Part model, mm, in its own coordinate system. A direction names the side the tool comes from. Round coordinates to 2 decimals unless told otherwise and drop trailing zeros. Write each loop counter-clockwise with the first axis right and the second up, starting at its lowest first coordinate (ties: lowest second). Pieces come first, ordered by that corner, then holes. Notation, with made-up numbers: M -32,71.25 L -11,71.25 A11 cw -11,86.25 Z; hole C 73.25,-10 d9. An arc over 180 degrees is marked long. Answer as a JSON object with one key per item and string values. Group by question number.
1. Two-plate mould, pull along Y, no slides. Class faces 1 (the face through (28, 4.75, -31)), 2 (the face through (57, 8, -10)), 3 (the face through (11.07, 6.34, -19.08)): +Y half, -Y half, draft (parallel to the pull), parting line (faces both ways), or undercut.
2. Band-saw the part on B-B, the plane z = -17.5. Write the cut outline in (x, y), plus the area to 3 significant figures.
3. Drop flat-ended pins along their axis: pin 1 (2.5 mm diameter, centred on x = 27.52, z = -32.31, fed in from +Y); pin 2 (2 mm diameter, centred on x = 39.5, y = 5.5, fed in from +Z); pin 3 (4 mm diameter, centred on x = 28, z = -31.5, fed in from +Y); pin 4 (2 mm diameter, centred on x = 44, z = -13.5, fed in from +Y). Give the stop position or say it passes through.
4. Band-saw the part on C-C, the plane z = -25. Write the cut outline in (x, y), plus the area to 3 significant figures.
5. Which spindle directions (+Z, -Z, +X, -X, +Y, -Y) get a long thin tool onto all of the face, cutting with end or side? Do faces 4 (the face through (30, 4.75, -18)), 5 (the face through (-1.15, 8.83, -4.93)), 6 (the face through (15.5, 6, -17)), 7 (the face through (28, 12, -35.17)). Say none if no direction does.
6. Drill centre lines: line 1 (X direction, y = 4, z = -27.5); line 2 (X direction, y = 6.5, z = -27.5); line 3 (X direction, y = 4.25, z = -15). Where is each one in solid material? Low to high. Write a range as from..to.
7. Band-saw the part on A-A, the plane x = 8.5. Write the cut outline in (y, z), plus the area to 3 significant figures.
8. Band-saw the part on D-D, the plane x = 54. Write the cut outline in (y, z), plus the area to 3 significant figures.
from build123d import *

# Parameters (mm, degrees)
SKETCH1_W                            = 55
SKETCH1_H                            = 42.17
BOSS_EXTRUDE1_DEPTH                  = 12.5
SKETCH2_W                            = 55
SKETCH2_H                            = 7
BOSS_EXTRUDE2_DEPTH                  = 2.5
SKETCH3_W                            = 16.25
SKETCH3_H                            = 35.17
CUT_EXTRUDE1_DEPTH                   = 7.25
CUT_EXTRUDE2_DEPTH                   = 71.424135777
SKETCH5_R                            = 2.85
SKETCH5_R_2                          = 2.35
CUT_EXTRUDE3_DEPTH                   = 0.5
SKETCH7_R                            = 5
BOSS_EXTRUDE3_DEPTH                  = 4
TAP_DRILL_FOR_10_32_TAP1_D           = 4.0386
TAP_DRILL_FOR_10_32_TAP1_DEPTH       = 4
TAP_DRILL_FOR_10_32_TAP1_CSINK_D     = 5.3086
TAP_DRILL_FOR_10_32_TAP1_CSINK_ANGLE = 90
TAP_DRILL_FOR_10_32_TAP1_TIP         = 1.213317848
SKETCH11_R                           = 1
CUT_EXTRUDE4_DEPTH                   = 71.059770197
TAP_DRILL_FOR_M3X0_5_TAP1_D          = 2.5
SKETCH15_R                           = 1.58
CUT_EXTRUDE5_DEPTH                   = 72.242956845
TAP_DRILL_FOR_M3X0_5_TAP3_D          = 2.5
TAP_DRILL_FOR_M3X0_5_TAP3_DEPTH      = 10
TAP_DRILL_FOR_M3X0_5_TAP3_TIP        = 0.751075774
BOSS_EXTRUDE4_DEPTH                  = 7
BOSS_EXTRUDE5_DEPTH                  = 7
SKETCH24_R                           = 1.58
CUT_EXTRUDE6_DEPTH                   = 10
TAP_DRILL_FOR_M3X0_5_TAP2_D          = 2.5


with BuildPart() as part:
    # Sketch1 → Boss-Extrude1 (new body)
    with BuildSketch(Plane(origin=(0, 0, 0), x_dir=(1, 0, 0), z_dir=(0, 1, 0))):
        with Locations((27.5, 21.085)):
            Rectangle(SKETCH1_W, SKETCH1_H)
    extrude(amount=BOSS_EXTRUDE1_DEPTH)

    # Sketch2 → Boss-Extrude2 (add)
    with BuildSketch(Plane(origin=(0, 12.5, 0), x_dir=(1, 0, 0), z_dir=(0, 1, 0))):
        with Locations((27.5, 38.67)):
            Rectangle(SKETCH2_W, SKETCH2_H)
    extrude(amount=BOSS_EXTRUDE2_DEPTH)

    # Sketch3 → Cut-Extrude1 (cut)
    with BuildSketch(Plane(origin=(0, 12.5, 0), x_dir=(1, 0, 0), z_dir=(0, 1, 0))):
        with Locations((25.465, 17.585)):
            Rectangle(SKETCH3_W, SKETCH3_H)
    extrude(amount=-CUT_EXTRUDE1_DEPTH, mode=Mode.SUBTRACT)

    # Sketch4 → Cut-Extrude2 (cut, through all)
    with BuildSketch(Plane(origin=(0, 12.5, 0), x_dir=(1, 0, 0), z_dir=(0, 1, 0))):
        with BuildLine():
            Line((15.5, 3.917342747), (15.5, 30.917342747))
            ThreePointArc((15.5, 30.917342747), (15.792893219, 31.624449528), (16.5, 31.917342747))
            Line((16.5, 31.917342747), (19.34, 31.917342747))
            ThreePointArc((19.34, 31.917342747), (20.047106781, 31.624449528), (20.34, 30.917342747))
            Line((20.34, 30.917342747), (20.34, 3.917342747))
            ThreePointArc((20.34, 3.917342747), (20.047106781, 3.210235966), (19.34, 2.917342747))
            Line((19.34, 2.917342747), (16.5, 2.917342747))
            ThreePointArc((16.5, 2.917342747), (15.792893219, 3.210235966), (15.5, 3.917342747))
        make_face()
    extrude(amount=-CUT_EXTRUDE2_DEPTH, mode=Mode.SUBTRACT)

    # Sketch5 → Cut-Extrude3 (cut)
    with BuildSketch(Plane(origin=(0, 5.25, 0), x_dir=(1, 0, 0), z_dir=(0, 1, 0))):
        with Locations(Location((24.34, 4.307342747, 0), (0, 0, 270))):
            Circle(SKETCH5_R)
        with Locations(Location((26.34, 11.307342747, 0), (0, 0, 270))):
            Circle(SKETCH5_R)
        with Locations(Location((29.84, 18.307342747, 0), (0, 0, 270))):
            Circle(SKETCH5_R)
        with Locations(Location((23.84, 25.307342747, 0), (0, 0, 270))):
            Circle(SKETCH5_R)
        with Locations(Location((27.52, 32.307342747, 0), (0, 0, 270))):
            Circle(SKETCH5_R_2)
    extrude(amount=-CUT_EXTRUDE3_DEPTH, mode=Mode.SUBTRACT)

    # Sketch7 → Boss-Extrude3 (add)
    with BuildSketch(Plane.XZ):
        with Locations(Location((27.52, -32.307342747, 0), (0, 0, 270))):
            Circle(SKETCH7_R)
    extrude(amount=BOSS_EXTRUDE3_DEPTH)

    # Tap Drill for #10-32 Tap1
    with Locations(Plane(origin=(0, -4, 0), x_dir=(-1, 0, 0), z_dir=(0, -1, 0))):
        with Locations((-27.52, 32.307342747)):
            CounterSinkHole(TAP_DRILL_FOR_10_32_TAP1_D / 2, TAP_DRILL_FOR_10_32_TAP1_CSINK_D / 2, depth=TAP_DRILL_FOR_10_32_TAP1_DEPTH, counter_sink_angle=TAP_DRILL_FOR_10_32_TAP1_CSINK_ANGLE)
            with Locations((0, 0, -(TAP_DRILL_FOR_10_32_TAP1_DEPTH + TAP_DRILL_FOR_10_32_TAP1_TIP / 2))):  # 118° drill point
                Cone(0, TAP_DRILL_FOR_10_32_TAP1_D / 2, TAP_DRILL_FOR_10_32_TAP1_TIP, mode=Mode.SUBTRACT)

    # Sketch11 → Cut-Extrude4 (cut, through all)
    with BuildSketch(Plane(origin=(0, 4.75, 0), x_dir=(1, 0, 0), z_dir=(0, 1, 0))):
        with Locations(Location((27.52, 32.307342747, 0), (0, 0, 270))):
            Circle(SKETCH11_R)
    extrude(amount=-CUT_EXTRUDE4_DEPTH, mode=Mode.SUBTRACT)

    # Tap Drill for M3x0.5 Tap1 (through all)
    with Locations(Plane(origin=(0, 12.5, 0), x_dir=(1, 0, 0), z_dir=(0, 1, 0))):
        with Locations((8.5, 7.5), (8.5, 27.5), (46.5, 27.5), (46.5, 7.5)):
            Hole(TAP_DRILL_FOR_M3X0_5_TAP1_D / 2)

    # Sketch15 → Cut-Extrude5 (cut, through all)
    with BuildSketch(Plane(origin=(0, 12.5, 0), x_dir=(1, 0, 0), z_dir=(0, 1, 0))):
        with Locations(Location((11, 17.5, 0), (0, 0, 270))):
            Circle(SKETCH15_R)
        with Locations(Location((44, 17.5, 0), (0, 0, 270))):
            Circle(SKETCH15_R)
    extrude(amount=-CUT_EXTRUDE5_DEPTH, mode=Mode.SUBTRACT)

    # Tap Drill for M3x0.5 Tap3
    with Locations(Plane.XY):
        with Locations((4, 7.5), (51, 7.5)):
            Hole(TAP_DRILL_FOR_M3X0_5_TAP3_D / 2, depth=TAP_DRILL_FOR_M3X0_5_TAP3_DEPTH)
            with Locations((0, 0, -(TAP_DRILL_FOR_M3X0_5_TAP3_DEPTH + TAP_DRILL_FOR_M3X0_5_TAP3_TIP / 2))):  # 118° drill point
                Cone(0, TAP_DRILL_FOR_M3X0_5_TAP3_D / 2, TAP_DRILL_FOR_M3X0_5_TAP3_TIP, mode=Mode.SUBTRACT)

    # Sketch22 → Boss-Extrude4 (add)
    with BuildSketch(Plane(origin=(55, 0, 0), x_dir=(0, 0, -1), z_dir=(1, 0, 0))):
        Polygon((0, 0), (42.17, 0), (42.17, 15), (35.17, 15), (35.17, 12.5), (0, 12.5), align=None)
    extrude(amount=BOSS_EXTRUDE4_DEPTH)

    # Sketch23 → Boss-Extrude5 (add)
    with BuildSketch(Plane.ZY):
        Polygon((0, 0), (0, 12.5), (-35.17, 12.5), (-35.17, 15), (-42.17, 15), (-42.17, 0), align=None)
    extrude(amount=BOSS_EXTRUDE5_DEPTH)

    # Sketch24 → Cut-Extrude6 (cut)
    with BuildSketch(Plane.XY):
        with Locations((57, 7.5)):
            Circle(SKETCH24_R)
        with Locations((-2, 7.5)):
            Circle(SKETCH24_R)
    extrude(amount=-CUT_EXTRUDE6_DEPTH, mode=Mode.SUBTRACT)

    # Tap Drill for M3x0.5 Tap2 (through all)
    with Locations(Plane(origin=(0, 15, 0), x_dir=(1, 0, 0), z_dir=(0, 1, 0))):
        with Locations((-3.5, 38.67), (58.5, 38.67)):
            Hole(TAP_DRILL_FOR_M3X0_5_TAP2_D / 2)


solid = part.part
Worked answers:
{
 "1": {"face 1": "+Y half", "face 2": "undercut", "face 3": "draft"},
 "2": {"outline": "M -7,0 L 9.42,0 L 9.42,12.5 L -7,12.5 Z; M 12.58,0 L 15.5,0 L 15.5,12.5 L 12.58,12.5 Z; M 20.34,0 L 42.42,0 L 42.42,12.5 L 33.59,12.5 L 33.59,5.25 L 32.57,5.25 L 32.57,4.75 L 27.11,4.75 L 27.11,5.25 L 20.34,5.25 Z; M 45.58,0 L 62,0 L 62,12.5 L 45.58,12.5 Z", "area": "624 mm^2"},
 "3": {"pin 1": "stops at y = 4.75", "pin 2": "stops at z = 0", "pin 3": "stops at y = 5.25", "pin 4": "stops at y = 12.5"},
 "4": {"outline": "M -7,0 L 15.5,0 L 15.5,12.5 L -7,12.5 Z; M 20.34,0 L 62,0 L 62,12.5 L 33.59,12.5 L 33.59,5.25 L 26.67,5.25 L 26.67,4.75 L 21.01,4.75 L 21.01,5.25 L 20.34,5.25 Z", "area": "703 mm^2"},
 "5": {"face 4": "+Y", "face 5": "+Z", "face 6": "+Y, -Y", "face 7": "+Z, +Y"},
 "6": {"line 1": "x = -7..7.25, 9.75..15.5, 20.34..45.25, 47.75..62", "line 2": "x = -7..7.25, 9.75..15.5, 33.59..45.25, 47.75..62", "line 3": "x = -7..15.5, 20.34..62"},
 "7": {"outline": "M 0,-42.17 L 15,-42.17 L 15,-35.17 L 12.5,-35.17 L 12.5,-28.75 L 0,-28.75 Z; M 0,-26.25 L 12.5,-26.25 L 12.5,-8.75 L 0,-8.75 Z; M 0,-6.25 L 12.5,-6.25 L 12.5,0 L 0,0 Z", "area": "482 mm^2"},
 "8": {"outline": "M 0,-42.17 L 15,-42.17 L 15,-35.17 L 12.5,-35.17 L 12.5,0 L 0,0 Z", "area": "545 mm^2"}
}
